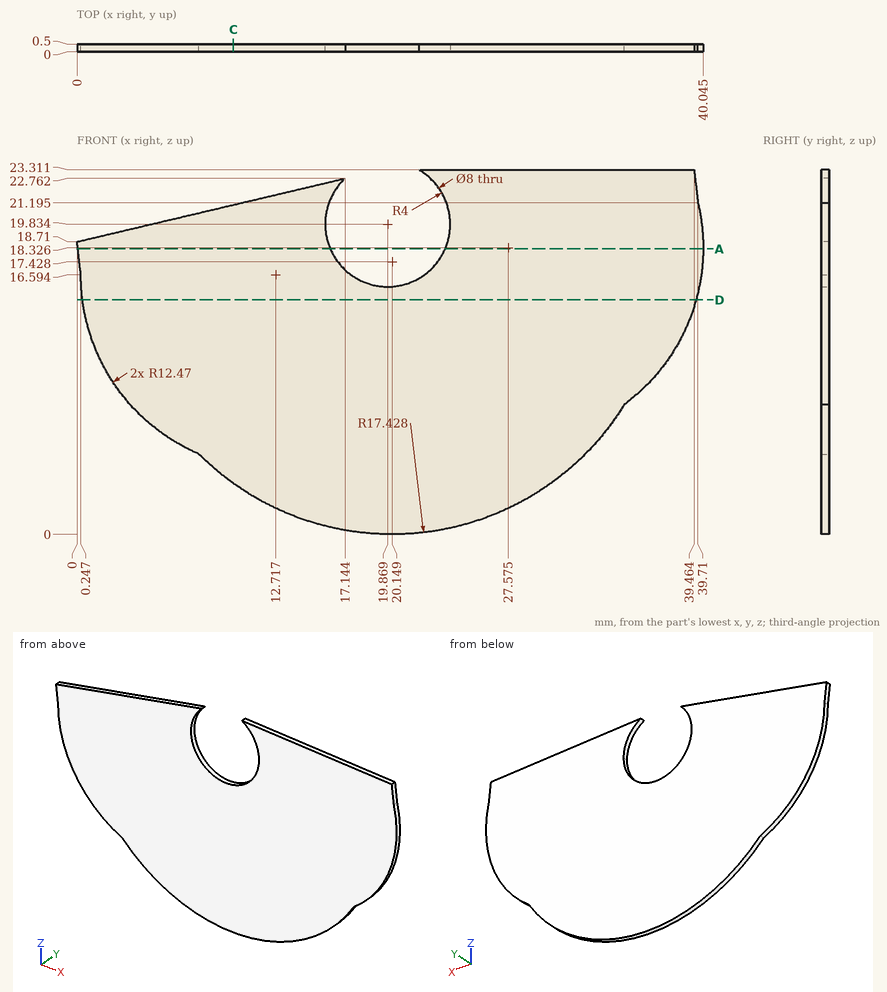
Check sheet for the drawn part. Datum: minimum x, y, z corner. Units: mm. Coordinates: 2 decimals unless noted, no trailing zeros. Loops run counter-clockwise (first coordinate to the right, second up) from the corner with the lowest first, then second, coordinate; pieces in that order, holes last. Notation, with made-up numbers: (-5, 77) - (14, 77) arc R16 ccw to (14, 89) - close; hole circle Ø7 at (-30, 58). An arc over 180 degrees is marked (long way). Put each result on its own line as item: value.
Item 1: Section check A-A (z = 18.25). Enter the section's corners in (x, y) (1 decimal).
Conclusion:
outline: (0.1, 0) - (16.2, 0) - (16.2, 0.5) - (0.1, 0.5) - close; (23.5, 0) - (40, 0) - (40, 0.5) - (23.5, 0.5) - close
Item 2: Gauge pin test, flat end, axial feed: pin 1 Ø5 at (x, z) = (7.5, 7.5) entering from -Y. Record the tip position at first contact, or that the pin passes through.
Conclusion:
pin 1: stops at y = 0
Item 3: Scan lines: line 1 along Z through (x, y) = (20, 0.1); line 2 along X through (y, z) = (0.3, 17) (1 decimal); line 3 along X through (y, z) = (0.15, 3) (1 decimal). Record each from-to range of solid material in increasing order.
Conclusion:
line 1: z = 0 to 15.84
line 2: x = 0.2 to 17, 22.7 to 40
line 3: x = 10.4 to 29.9
Item 4: Section check C-C (x = 10). Enter the section's corners in (y, z).
Conclusion:
outline: (0, 3.26) - (0.5, 3.26) - (0.5, 21.07) - (0, 21.07) - close
Item 5: Section check D-D (z = 15). Enter the section's corners in (x, y).
Conclusion:
outline: (0.35, 0) - (39.59, 0) - (39.59, 0.5) - (0.35, 0.5) - close
